from build123d import *

# Parameters (mm, degrees)
F1_DEPTH      = 25.146
F1_DEPTH_BACK = 25.4
F2_R          = 12.7
F3_R          = 25.4
F4_W          = 43.2194133058
F4_H          = 25.146
F5_DEPTH      = 25.4


with BuildPart() as f1:
    # F0 (on Front) → F1 (new body, two sides)
    with BuildSketch(Plane.XZ) as f1_sk:
        Polygon((-59.228181839, 16.3945462555), (-59.228181839, -22.3981812596), (67.3100054264, -19.8581814766), (58.5354566574, 33.9436382055), (15.12454357, 53.1090945005), (-31.5190926194, 41.7945459485), align=None)
    extrude(amount=F1_DEPTH)
    extrude(f1_sk.sketch, amount=-F1_DEPTH_BACK)

    # F2
    f2_edges = [f1.edges().sort_by_distance(p)[0] for p in [
        (58.535457, 0.127, 33.943638),
    ]]
    fillet(f2_edges, radius=F2_R)

    # F3
    f3_edges = [f1.edges().sort_by_distance(p)[0] for p in [
        (-31.519093, 0.127, 41.794546),
        (15.124544, 0.127, 53.109095),
    ]]
    fillet(f3_edges, radius=F3_R)

    # F4 (on face) → F5 (cut)
    with BuildSketch(Plane(origin=(0.4255624903, 0, -21.200752239), x_dir=(0.9997985984, 0, 0.0200689474), z_dir=(0.0200689474, 0, -0.9997985984))):
        with Locations((3.2696425915, -0.127)):
            Rectangle(F4_W, F4_H)
    extrude(amount=-F5_DEPTH, mode=Mode.SUBTRACT)


solid = f1.part
Could you check a few things on this model? Use its own coordinates, in mm. Coordinates: 2 decimals unless noted, no trailing zeros. Loops run counter-clockwise (first coordinate to the right, second up) from the corner with the lowest first, then second, coordinate; pieces in that order, holes last.
1. Imagine slicing it at D-D (z = -5). Please give me the cut outline in (x, y), and give its area (3 significant figures).
2. Imagine slicing it at B-B (z = -15). Please give me the cut outline in (x, y).
3. Imagine slicing it at C-C (x = 10). Please give me the cut outline in (y, z), and give its area (3 significant figures).
4. We'd pull the mould along Y, two halves only. Please class faces 1 (the face through (3, 12.7, -9)), 2 (the face through (-8.98, -0.23, 47.26)), 3 (the face through (3, 25.4, 7)): released by +Y, released by -Y, zero draft, split by the parting line, or undercut.
5. I need wall thicknesses on L1, parallel to Y at x = 6, z = -10; L2, parallel to X at y = -8, z = -13.5; L3, parallel to Z at x = 56, y = 5.5. Which ranges of each line are inside material? Lowest first, please.
6. For P1, Ø12, axis at y = 8, z = 37.5, coming from the +X side; P2, Ø6, axis at y = -17.5, z = -12, coming from the +X side; P3, Ø6, axis at y = -11.5, z = 35, coming from the -X side, each with a flat end and sliding along its axis, tell me the tip position at first contact or that it passes through.
7. Imagine slicing it at A-A (y = -10.5). Please give me the cut outline in (x, z).
Computed values:
1. outline: (-59.23, -25.15) - (64.89, -25.15) - (64.89, 25.4) - (-59.23, 25.4) - close; hole (-18.24, -12.45) - (24.98, -12.45) - (24.98, 12.7) - (-18.24, 12.7) - close
1. area: 5,190 mm2
2. outline: (-59.23, -25.15) - (66.52, -25.15) - (66.52, 25.4) - (-59.23, 25.4) - close; hole (-18.04, -12.45) - (25.19, -12.45) - (25.19, 12.7) - (-18.04, 12.7) - close
3. outline: (-25.15, -21.01) - (-12.45, -21.01) - (-12.45, 4.4) - (12.7, 4.4) - (12.7, -21.01) - (25.4, -21.01) - (25.4, 51.65) - (-25.15, 51.65) - close
3. area: 3,030 mm2
4. face 1: undercut
4. face 2: zero draft
4. face 3: released by +Y
5. L1: y = -25.15 to -12.45, 12.7 to 25.4
5. L2: x = -59.23 to -18.07, 25.16 to 66.27
5. L3: z = -20.09 to 34.17
6. P1: stops at x = 58.08
6. P2: stops at x = 66.52
6. P3: stops at x = -42.2
7. outline: (-59.23, -22.4) - (-17.91, -21.57) - (-18.42, 3.83) - (24.79, 4.69) - (25.3, -20.7) - (67.31, -19.86) - (59.64, 27.15) arc R12.7 ccw to (52.24, 36.72) - (23, 49.63) arc R25.4 ccw to (6.76, 51.08) - (-25.16, 43.34) arc R25.4 ccw to (-36.34, 37.38) - (-59.23, 16.39) - close
